from build123d import *

# Parameters (mm, degrees)
BOSS_EXTRUDE1_DEPTH = 44.449999999999996
BOSS_EXTRUDE2_START = 12.7
SKETCH2_R           = 127.00000000000026
SKETCH2_R_2         = 38.09999999999998
SKETCH2_R_3         = 152.39999999999995
SKETCH2_R_4         = 38.10000000000004
SKETCH2_R_5         = 127.00000000000524
SKETCH2_R_6         = 38.10000000000009
SKETCH2_R_7         = 101.59999999999945
SKETCH2_R_8         = 38.10000000000007
BOSS_EXTRUDE2_DEPTH = 12.7


with BuildPart() as part:
    # Sketch1 → Boss-Extrude1 (new, symmetric)
    with BuildSketch(Plane(origin=(0, 0, 0), x_dir=(0, 0, -1), z_dir=(1, 0, 0))):
        with BuildLine():
            Line((292.75767615040746, -1.5786e-13), (864.2576761504075, -4.1113e-13))
            ThreePointArc((864.2576761504075, -4.1113e-13), (1190.1025822900356, 94.39396631749571), (1415.036093761449, 348.34285714285653))
            Line((1415.036093761449, 348.34285714285653), (1656.0016514662793, 856.3428571428565))
            ThreePointArc((1656.0016514662793, 856.3428571428565), (1800.5110136275975, 899.6556499579777), (1828.8000000000002, 751.4710116727003))
            ThreePointArc((1828.8000000000002, 751.4710116727003), (1614.8079841790877, 177.34138113633213), (1751.9712010597207, -419.8216346557389))
            ThreePointArc((1751.9712010597207, -419.8216346557389), (1715.4290562941019, -585.9160522435095), (1546.4465674603723, -566.7430930182793))
            ThreePointArc((1546.4465674603723, -566.7430930182793), (1067.265507093057, -350.8585161091587), (588.0844467257416, -566.7430930182793))
            ThreePointArc((588.0844467257416, -566.7430930182793), (485.76498042432655, -609.3961073308187), (388.92622108801334, -555.4442074165836))
            Line((388.92622108801334, -555.4442074165836), (167.91890460076553, -239.8130488999002))
            ThreePointArc((167.91890460076553, -239.8130488999002), (157.5772251740463, -82.02951134298137), (292.75767615040746, -1.5786e-13))
        make_face()
        with BuildLine():
            Line((292.7576761504074, -50.8), (864.2576761504075, -50.8))
            ThreePointArc((864.2576761504075, -50.8), (1217.2563244683374, 51.46013017728751), (1460.9342952290358, 326.571428571428))
            Line((1460.9342952290358, 326.571428571428), (1701.8998529338662, 834.571428571428))
            ThreePointArc((1701.8998529338662, 834.571428571428), (1774.1545340145256, 856.2278249789883), (1788.2990272007264, 782.1355058363492))
            ThreePointArc((1788.2990272007264, 782.1355058363492), (1564.1169153883338, 180.66636908396612), (1707.8117140251866, -444.93298079344424))
            ThreePointArc((1707.8117140251866, -444.93298079344424), (1685.8864271658267, -544.589631346108), (1584.4969338655828, -533.0858558109679))
            ThreePointArc((1584.4969338655828, -533.0858558109679), (1067.265507093057, -300.058516109159), (550.0340803205312, -533.0858558109682))
            ThreePointArc((550.0340803205312, -533.0858558109682), (488.6424005396823, -558.6776643984912), (430.53914493789466, -526.306524449951))
            Line((430.53914493789466, -526.306524449951), (209.53182845064617, -210.6753659332667))
            ThreePointArc((209.53182845064617, -210.6753659332667), (202.6373754995001, -105.48634089532098), (292.7576761504074, -50.8))
        make_face(mode=Mode.SUBTRACT)
    extrude(amount=BOSS_EXTRUDE1_DEPTH, both=True)

    # Sketch2 → Boss-Extrude2 (add)
    # profile 1 of 4: a face of its own
    with BuildSketch(Plane(origin=(44.449999999999996, 0, 0), x_dir=(0, 0, -1), z_dir=(1, 0, 0)).offset(BOSS_EXTRUDE2_START)):
        with Locations((492.95853071271534, -482.60000000000036)):
            Circle(SKETCH2_R)
        with Locations((492.95853071271534, -482.60000000000036)):
            Circle(SKETCH2_R_2, mode=Mode.SUBTRACT)
    # profile 2 of 4: a face of its own
    with BuildSketch(Plane(origin=(44.449999999999996, 0, 0), x_dir=(0, 0, -1), z_dir=(1, 0, 0)).offset(BOSS_EXTRUDE2_START)):
        with Locations((292.7576761504074, -152.40000000000018)):
            Circle(SKETCH2_R_3)
        with Locations((292.7576761504074, -152.40000000000018)):
            Circle(SKETCH2_R_4, mode=Mode.SUBTRACT)
    # profile 3 of 4: a face of its own
    with BuildSketch(Plane(origin=(44.449999999999996, 0, 0), x_dir=(0, 0, -1), z_dir=(1, 0, 0)).offset(BOSS_EXTRUDE2_START)):
        with Locations((1641.5724834734083, -482.6000000000008)):
            Circle(SKETCH2_R_5)
        with Locations((1641.5724834734083, -482.6000000000008)):
            Circle(SKETCH2_R_6, mode=Mode.SUBTRACT)
    # profile 4 of 4: a face of its own
    with BuildSketch(Plane(origin=(44.449999999999996, 0, 0), x_dir=(0, 0, -1), z_dir=(1, 0, 0)).offset(BOSS_EXTRUDE2_START)):
        with Locations((1747.798054401453, 812.7999999999992)):
            Circle(SKETCH2_R_7)
        with Locations((1747.798054401453, 812.7999999999992)):
            Circle(SKETCH2_R_8, mode=Mode.SUBTRACT)
    boss_extrude2 = extrude(amount=-BOSS_EXTRUDE2_DEPTH)

    # Mirror1: Boss-Extrude2 across plane
    add(boss_extrude2.mirror(Plane(origin=(0, 0, 0), x_dir=(0, 0, 1), z_dir=(1, 0, 0))))


solid = part.part
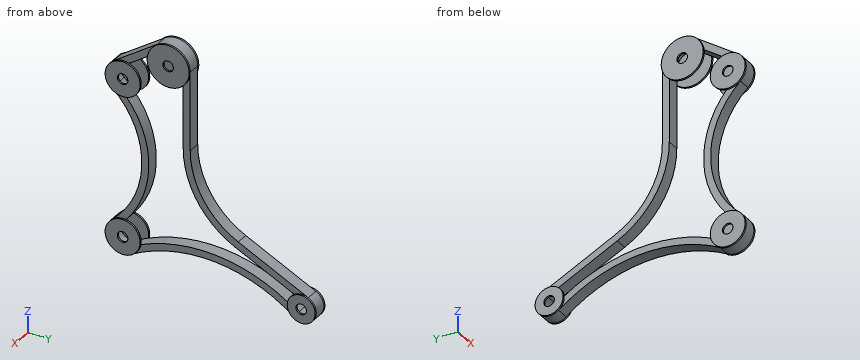
Part model, mm, in its own coordinate system. Give positions to 0.01 mm unless a question says otherwise; leave off trailing zeros. Write each loop counter-clockwise with the first axis right and the second up, starting at its lowest first coordinate (ties: lowest second). Pieces come first, ordered by that corner, then holes.
1) Cut at C-C on y = -152.4. Write the cut outline in (x, z), then the cut area to 3 significant figures.
Resolved:
outline: (-57.15, -445.16) - (-44.45, -445.16) - (-44.45, -330.86) - (-57.15, -330.86) - close; (-57.15, -254.66) - (-44.45, -254.66) - (-44.45, -191.16) - (44.45, -191.16) - (44.45, -254.66) - (57.15, -254.66) - (57.15, -140.36) - (-57.15, -140.36) - close; (-44.45, -1644.67) - (44.45, -1644.67) - (44.45, -1592.36) - (-44.45, -1592.36) - close; (44.45, -445.16) - (57.15, -445.16) - (57.15, -330.86) - (44.45, -330.86) - close
area: 15,000 mm2
2) Cut at B-B on x = 25. Write the cut outline in (y, z), then the cut area to 3 significant figures.
Resolved:
outline: (-566.74, -1546.45) arc R127 ccw to (-419.82, -1751.97) arc R1066.8 cw to (751.47, -1828.8) arc R101.6 ccw (long way) to (856.34, -1656) - (348.34, -1415.04) arc R609.6 cw to (0, -864.26) - (0, -292.76) arc R152.4 ccw to (-239.81, -167.92) - (-555.44, -388.93) arc R127 ccw to (-566.74, -588.08) arc R639.74 cw to start; hole (-533.09, -1584.5) arc R76.2 ccw to (-444.93, -1707.81) arc R1117.6 cw to (782.14, -1788.3) arc R50.8 ccw (long way) to (834.57, -1701.9) - (326.57, -1460.93) arc R660.4 cw to (-50.8, -864.26) - (-50.8, -292.76) arc R101.6 ccw to (-210.68, -209.53) - (-526.31, -430.54) arc R76.2 ccw to (-533.09, -550.03) arc R690.54 cw to start
area: 287,000 mm2
3) Pin check, flat tips, straight feed: pin 1 (1.5 mm diameter, centred on x = -28.5, y = -413, fed in from +Z); pin 2 (6 mm diameter, centred on x = -12, y = -413.5, fed in from +Z); pin 3 (10 mm diameter, centred on x = 32.5, z = -558.5, fed in from -Y). Stop position of each tip, or through.
Resolved:
pin 1: stops at z = -288.66
pin 2: stops at z = -287.44
pin 3: stops at y = -594.24
4) Cut at D-D on y = 616.5. Write the cut outline in (x, z).
Resolved:
outline: (-44.45, -1741.77) - (44.45, -1741.77) - (44.45, -1684.35) - (-44.45, -1684.35) - close; (-44.45, -1598.46) - (44.45, -1598.46) - (44.45, -1542.23) - (-44.45, -1542.23) - close
5) Cut at A-A on y = 812.8. Write the cut outline in (x, z).
Resolved:
outline: (-57.15, -1849.4) - (57.15, -1849.4) - (57.15, -1785.9) - (44.45, -1785.9) - (44.45, -1798.6) - (-44.45, -1798.6) - (-44.45, -1785.9) - (-57.15, -1785.9) - close; (-57.15, -1709.7) - (-44.45, -1709.7) - (-44.45, -1691.57) - (44.45, -1691.57) - (44.45, -1709.7) - (57.15, -1709.7) - (57.15, -1646.2) - (44.45, -1646.2) - (44.45, -1635.35) - (-44.45, -1635.35) - (-44.45, -1646.2) - (-57.15, -1646.2) - close
6) Probe L1, parallel to Z at x = 48.5, y = -482.6; L2, parallel to Z at x = -51, y = -484; L3, parallel to Z at x = 48, y = 812. List the from-to ranges inside material, lowest first.
Resolved:
L1: z = -1768.57 to -1679.67, -1603.47 to -1514.57, -619.96 to -531.06, -454.86 to -365.96
L2: z = -1768.56 to -1679.65, -1603.5 to -1514.58, -619.95 to -531.03, -454.88 to -365.97
L3: z = -1849.39 to -1785.89, -1709.71 to -1646.2
